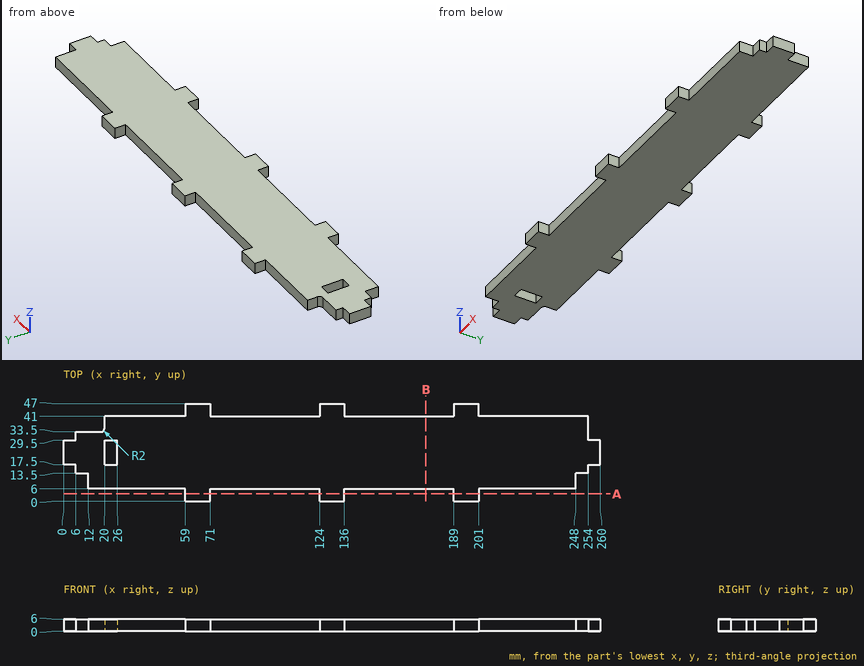
Design review of the part shown in the three views and the two pictorial views. Dimensions are in mm from the part's minimum x, y and z. Give positions to 0.01 mm unless a question says otherwise; leave off trailing zeros. Write each loop counter-clockwise with the first axis right and the second up, starting at its lowest first coordinate (ties: lowest second). Pieces come first, ordered by that corner, then holes.
Item 1: Wall thickness on probe 1 along X at (y, z) = (42.5, 4.8); probe 2 along X at (y, z) = (24, 4.35); probe 3 along Y at (x, z) = (49.5, 4.55): over which ranges is each line inside the solid? List them lowest first.
Item 2: Insertion check: P1, Ø1.5, axis at x = 100, z = 3, coming from the -Y side; P2, Ø1.8, axis at x = 7.5, z = 2.5, coming from the -Y side; P3, Ø1.8, axis at y = 43, z = 3, coming from the -X side. Each pin has a flat end and moves straight along its axis. Give the tip position at first contact, or say it passes through.
Item 3: Take a section at A-A (y = 3.5). Give the boundary of the cut face in (x, z).
Item 4: Take a section at B-B (x = 175.5). Give the boundary of the cut face in (y, z).
Established:
1. probe 1: x = 59 to 71, 124 to 136, 189 to 201
1. probe 2: x = 0 to 20, 26 to 260
1. probe 3: y = 6 to 41
2. P1: stops at y = 6
2. P2: stops at y = 13.5
2. P3: stops at x = 59
3. outline: (59, 0) - (71, 0) - (71, 6) - (59, 6) - close; (124, 0) - (136, 0) - (136, 6) - (124, 6) - close; (189, 0) - (201, 0) - (201, 6) - (189, 6) - close
4. outline: (6, 0) - (41, 0) - (41, 6) - (6, 6) - close
